from build123d import *

# Parameters (mm, degrees)
SZKIC2_W                    = 32
SZKIC2_H                    = 67
SZKIC2_R                    = 1.375000051
SZKIC2_R_2                  = 1.375001066
SZKIC2_R_3                  = 1.375000054
SZKIC2_R_4                  = 1.374997602
SZKIC2_W_2                  = 5
DODANIE_WYCI_GNI_CIE1_DEPTH = 4
SZKIC7_W                    = 20
SZKIC7_H                    = 7.5
DODANIE_WYCI_GNI_CIE2_DEPTH = 4


with BuildPart() as part:
    # Szkic2 → Dodanie-wyciągnięcie1 (new body)
    # profile 1 of 2: a face of its own
    with BuildSketch(Plane.XY):
        with Locations((16, 33.5)):
            Rectangle(SZKIC2_W, SZKIC2_H)
        with Locations((4.59999689, 4.59999658)):
            Circle(SZKIC2_R, mode=Mode.SUBTRACT)
        with Locations((27.600003502, 4.59999658)):
            Circle(SZKIC2_R_2, mode=Mode.SUBTRACT)
        with Locations((4.600005213, 62.599996076)):
            Circle(SZKIC2_R_3, mode=Mode.SUBTRACT)
        with Locations((27.600003502, 62.599996076)):
            Circle(SZKIC2_R_4, mode=Mode.SUBTRACT)
    # profile 2 of 2: a face of its own
    with BuildSketch(Plane.XY):
        with Locations((34.5, 33.5)):
            Rectangle(SZKIC2_W_2, SZKIC2_H)
    extrude(amount=DODANIE_WYCI_GNI_CIE1_DEPTH)

    # Szkic7 → Dodanie-wyciągnięcie2 (add)
    with BuildSketch(Plane(origin=(37, 0, 0), x_dir=(0, 0, -1), z_dir=(1, 0, 0))):
        with Locations((-14, 3.75)):
            Rectangle(SZKIC7_W, SZKIC7_H)
        with Locations((10, 3.75)):
            Rectangle(SZKIC7_W, SZKIC7_H)
        with Locations((-14, 63.25)):
            Rectangle(SZKIC7_W, SZKIC7_H)
        with Locations((10, 63.25)):
            Rectangle(SZKIC7_W, SZKIC7_H)
    extrude(amount=-DODANIE_WYCI_GNI_CIE2_DEPTH)


solid = part.part
Part model, mm, in its own coordinate system. A direction names the side the tool comes from. Coordinates: 2 decimals unless noted, no trailing zeros. Order: outer loops, then holes, each group sorted by start corner. A loop starts at its lowest first (then second) coordinate and runs counter-clockwise, first axis right, second up. Notation, with made-up numbers: (29, 10) - (41, 10) arc R20 ccw to (41, 35) - close; hole circle Ø4 at (16, 55.25). An arc over 180 degrees is marked (long way). Use CSV: the item, a comma, the result in double quotes.
Item 1: Probe probe 1 along Z at (x, y) = (26, 25); probe 2 along Y at (x, z) = (34, -10); probe 3 along X at (y, z) = (6, -4.5). List the from-to ranges inside material, lowest first.
Solved:
probe 1,"z = 0 to 4"
probe 2,"y = 0 to 7.5, 59.5 to 67"
probe 3,"x = 33 to 37"
Item 2: Saw through at A-A on z = 10. Give the cut face in (x, y).
Solved:
outline,"(33, 0) - (37, 0) - (37, 7.5) - (33, 7.5) - close; (33, 59.5) - (37, 59.5) - (37, 67) - (33, 67) - close"
Item 3: Mould opens along X. For faces 5 (the face through (27.3, 61.26, 1.97)), 6 (the face through (27, 67, 2)), 7 (the face through (33, 4, -10)) say: +X half, -X half, draft (parallel to the pull), parting line (faces both ways), or undercut.
Solved:
face 5,"undercut"
face 6,"draft"
face 7,"-X half"
Item 4: Saw through at B-B on y = 56.5. Give the cut face in (x, z).
Solved:
outline,"(0, 0) - (37, 0) - (37, 4) - (0, 4) - close"
Item 5: 3-axis set-ups, long thin cutter, end or side, ignore diameter. For faces 1 (the face through (35, 59.5, 14)), 2 (the face through (33, 63, 14)), 3 (the face through (35, 7.5, -10)), 4 (the face through (33, 63, -10)): which of +Z, -Z, +X, -X, +Y, -Y reach the whole face in a straight line?
Solved:
face 1,"+Z, +X, -X"
face 2,"+Z, -X, +Y, -Y"
face 3,"-Z, +X, -X"
face 4,"-Z, -X, +Y, -Y"
Item 6: Saw through at C-C on x = 30. Give the cut face in (y, z).
Solved:
outline,"(0, 0) - (67, 0) - (67, 4) - (0, 4) - close"
Item 7: Drop flat-ended pins along their axis: P1, Ø8, axis at y = 4.5, z = 18, coming from the -X side; P2, Ø1.5, axis at y = 60, z = 2, coming from the -X side; P3, Ø1, axis at x = 13.5, y = 36, coming from the -Z side; P4, Ø18.5, axis at x = 26.5, y = 30, coming from the +Z side. Give the stop position or say it passes through.
Solved:
P1,"stops at x = 33"
P2,"stops at x = 0"
P3,"stops at z = 0"
P4,"stops at z = 4"
